Can you work these out from the model? Positions are in its coordinate system, mm. Give positions to 0.01 mm unless a question says otherwise; leave off trailing zeros. Loops run counter-clockwise (first coordinate to the right, second up) from the corner with the lowest first, then second, coordinate; pieces in that order, holes last. Notation, with made-up numbers: M 5,22 L 48,22 A27 cw 48,45 Z; hole C -20,44.25 d6. An arc over 180 degrees is marked long. Answer as a JSON object with one key per item and string values.
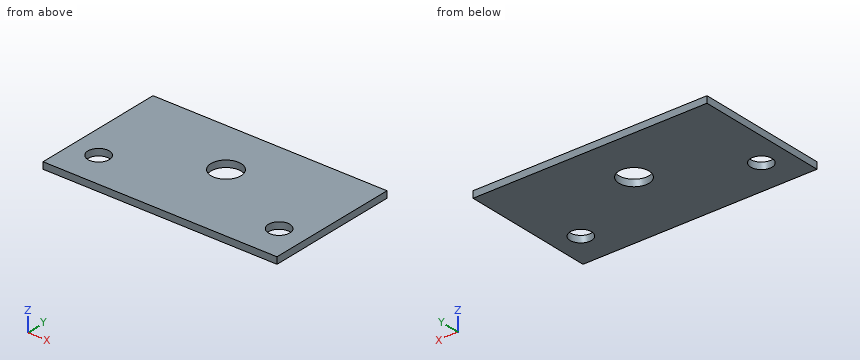
Autodesk Inventor part; units mm, degrees
ref_plane "YZ Plane" through (0, 0, 0) normal (1, 0, 0) x (0, 1, 0)
ref_plane "XZ Plane" through (0, 0, 0) normal (0, 1, 0) x (-1, 0, 0)
ref_plane "XY Plane" through (0, 0, 0) normal (0, 0, 1) x (1, 0, 0)
sketch "スケッチ1" plane through (0, 0, 0) normal (0, 0, 1) x (1, 0, 0)
  line L0 (0, 0) -> (35, 0)
  line L1 (35, 0) -> (35, 20)
  line L2 (35, 20) -> (0, 20)
  line L3 (0, 20) -> (0, 0)
  dimension "d0" = 20
  dimension "d1" = 35
extrude "押し出し1" add sketch "スケッチ1" along normal blind 1
sketch "スケッチ2" plane through (0, 0, 1) normal (0, 0, 1) x (1, 0, 0)
  line L0 (35, 20) -> (0, 20)
  point P0 (0, 0)
  point P1 (17.5, 12)
  point P2 (17.5, 20)
  dimension "d4" = 8
hole "穴1" at (17.5, 12, 1) direction (0, 0, -1) diameter 4.5 end through all
sketch "スケッチ3" plane through (0, 0, 1) normal (0, 0, 1) x (1, 0, 0)
  line L0 (0, 20) -> (0, 0)
  line L1 (0, 0) -> (35, 0)
  line L2 (35, 20) -> (0, 20)
  point P0 (4, 5.25)
  point P1 (31, 5.25)
  dimension "d12" = 27
  dimension "d13" = 4
  dimension "d22" = 14.75
hole "穴2" at (4, 5.25, 1) at (31, 5.25, 1) direction (0, 0, -1) diameter 3.2 end through all
properties part number "CLS_typeC_31.4N_plate"
1) Please list where these lines run through material, in increasing order: line 1 along X through (y, z) = (5.25, 0.8); line 2 along Y through (x, z) = (4, 0.35); line 3 along X through (y, z) = (4.75, 0.45). Write a range as from..to.
Answer list:
{"line 1": "0..2.4, 5.6..29.4, 32.6..35", "line 2": "0..3.65, 6.85..20", "line 3": "0..2.48, 5.52..29.48, 32.52..35"}
2) Suppose I cut it at C-C, the plane z = 0.3. Write out the boundary of the cut face in (x, y).
Answer list:
{"outline": "M 0,0 L 35,0 L 35,20 L 0,20 Z; hole C 4,5.25 d3.2; hole C 17.5,12 d4.5; hole C 31,5.25 d3.2"}
3) Suppose I cut it at B-B, the plane x = 31. Write out the boundary of the cut face in (y, z).
Answer list:
{"outline": "M 0,0 L 3.65,0 L 3.65,1 L 0,1 Z; M 6.85,0 L 20,0 L 20,1 L 6.85,1 Z"}
4) Will this pin go through, and if not, where does the flat tip stop? pin 1 Ø1.9 at (x, y) = (4, 5.25) entering from -Z.
Answer list:
{"pin 1": "through"}
5) Suppose I cut it at A-A, the plane y = 12. Write out the boundary of the cut face in (x, z).
Answer list:
{"outline": "M 0,0 L 15.25,0 L 15.25,1 L 0,1 Z; M 19.75,0 L 35,0 L 35,1 L 19.75,1 Z"}
6) Suppose I cut it at D-D, the plane y = 5.25. Write out the boundary of the cut face in (x, z).
Answer list:
{"outline": "M 0,0 L 2.4,0 L 2.4,1 L 0,1 Z; M 5.6,0 L 29.4,0 L 29.4,1 L 5.6,1 Z; M 32.6,0 L 35,0 L 35,1 L 32.6,1 Z"}
